Read the model definition and answer for the solid it produces. Units are mm, in the model's axes. Face numbers are marked on the shaded views. A direction names the side the tool comes from. Coordinates: 2 decimals unless noted, no trailing zeros. Write each loop counter-clockwise with the first axis right and the second up, starting at its lowest first coordinate (ties: lowest second). Pieces come first, ordered by that corner, then holes.
(1) Given pin 1 (6.5 mm diameter, centred on x = 13.5, y = 9.5, fed in from +Z); pin 2 (7.5 mm diameter, centred on x = 13, z = 9, fed in from -Y); pin 3 (2 mm diameter, centred on x = 12.5, z = 9.5, fed in from +Y), each flat-ended and moving along its own axis, determine where each tip first touches the part or whether it passes through.
(2) Section C-C on x = 12.5 is taken. Write down the section's boundary in (y, z).
(3) Section D-D on z = 0.5 is taken. Write down the section's boundary in (x, y), then the cut area to 3 significant figures.
(4) Which of the six approach directions +Z, -Z, +X, -X, +Y, -Y give full straight-line access (tool end or side, diameter ignored) to the marked faces 1, 2 and 3?
(5) Section B-B on y = 10.5 is taken. Write down the section's boundary in (x, z).
(6) Find the intervals of material crossed by probe 1 along X at (y, z) = (1.25, 10.5); probe 2 along Y at (x, z) = (7.5, 6); probe 3 along Y at (x, z) = (11.75, 0.5), in increasing order.
(7) Section A-A on z = 7.5 is taken. Write down the section's boundary in (x, y), then the cut area to 3 significant figures.
from build123d import *

# Parameters (mm, degrees)
F0_W      = 22
F0_H      = 15
F1_DEPTH  = 18
F2_T      = -1
F11_DEPTH = 25
F13_DEPTH = 25
F16_R     = 0.5
F17_DEPTH = 50
F20_DEPTH = 50


with BuildPart() as f1:
    # F0 (on Top) → F1 (new body)
    with BuildSketch(Plane.XY):
        with Locations((11, 7.5)):
            Rectangle(F0_W, F0_H)
    extrude(amount=F1_DEPTH)

    # F2
    f2_openings = [f1.faces().sort_by_distance(p)[0] for p in [
        (11, 7.5, 18),
    ]]
    offset(amount=F2_T, openings=f2_openings)

    # F5 (on offset) → F6 section 0
    with BuildSketch(Plane.XY.offset(-2.5)):
        Polygon((-0.5, 2), (-0.5, -0.5), (2, -0.5), (2, 0), (0, 0), (0, 2), align=None)
    # F3 (on face) → F6 section 1
    with BuildSketch(Plane(origin=(0, 0, 0), x_dir=(1, 0, 0), z_dir=(0, 0, -1))):
        Polygon((4, 0), (0, 0), (0, -4), (0.5, -4), (0.5, -0.5), (4, -0.5), align=None)
    loft()

    # F3 (on face) → F7 section 0
    with BuildSketch(Plane(origin=(0, 0, 0), x_dir=(1, 0, 0), z_dir=(0, 0, -1))):
        Polygon((0.5, -11), (0, -11), (0, -15), (4, -15), (4, -14.5), (0.5, -14.5), align=None)
    # F5 (on offset) → F7 section 1
    with BuildSketch(Plane.XY.offset(-2.5)):
        Polygon((-0.5, 13), (0, 13), (0, 15), (2, 15), (2, 15.5), (-0.5, 15.5), align=None)
    loft()

    # F3 (on face) → F8 section 0
    with BuildSketch(Plane(origin=(0, 0, 0), x_dir=(1, 0, 0), z_dir=(0, 0, -1))):
        Polygon((22, -15), (22, -11), (21.5, -11), (21.5, -14.5), (18, -14.5), (18, -15), align=None)
    # F5 (on offset) → F8 section 1
    with BuildSketch(Plane.XY.offset(-2.5)):
        Polygon((20, 15.5), (20, 15), (22, 15), (22, 13), (22.5, 13), (22.5, 15.5), align=None)
    loft()

    # F3 (on face) → F9 section 0
    with BuildSketch(Plane(origin=(0, 0, 0), x_dir=(1, 0, 0), z_dir=(0, 0, -1))):
        Polygon((22, 0), (18, 0), (18, -0.5), (21.5, -0.5), (21.5, -4), (22, -4), align=None)
    # F5 (on offset) → F9 section 1
    with BuildSketch(Plane.XY.offset(-2.5)):
        Polygon((22, 2), (22, 0), (20, 0), (20, -0.5), (22.5, -0.5), (22.5, 2), align=None)
    loft()

    # F10 (on face) → F11 (cut)
    with BuildSketch(Plane.XZ):
        Polygon((20, 15), (22, 15), (22, 18), (0, 18), (0, 15), (2, 15), (3.1547005384, 13), (18.8452994616, 13), align=None)
    extrude(amount=-F11_DEPTH, mode=Mode.SUBTRACT)

    # F12 (on face) → F13 (cut)
    with BuildSketch(Plane.YZ.offset(22)):
        Polygon((13, 15), (2, 15), (3.1547005384, 13), (11.8452994616, 13), align=None)
    extrude(amount=-F13_DEPTH, mode=Mode.SUBTRACT)

    # F16 (on face) → F17 (cut)
    with BuildSketch(Plane(origin=(22.0745514368, 14.8894729496, 0), x_dir=(-0.5591929035, 0.8290375726, 0), z_dir=(0.8290375726, 0.5591929035, 0))):
        with Locations((0.133319712, 14)):
            Circle(F16_R)
    extrude(amount=-F17_DEPTH, mode=Mode.SUBTRACT)

    # F19 (on face) → F20 (cut)
    with BuildSketch(Plane(origin=(15.1206725276, -10.1990224002, 0), x_dir=(0.5591929035, 0.8290375726, 0), z_dir=(0.8290375726, -0.5591929035, 0))):
        with BuildLine():
            ThreePointArc((12.8022438764, 14), (12.6557972669, 14.3535533906), (12.3022438764, 14.5))
            Line((12.3022438764, 14.5), (12.3022438764, 13.5))
            ThreePointArc((12.3022438764, 13.5), (12.6557972669, 13.6464466094), (12.8022438764, 14))
        make_face()
        with BuildLine():
            Line((12.3022438764, 13.5), (12.3022438764, 14.5))
            ThreePointArc((12.3022438764, 14.5), (11.8022438764, 14), (12.3022438764, 13.5))
        make_face()
    extrude(amount=-F20_DEPTH, mode=Mode.SUBTRACT)


solid = f1.part
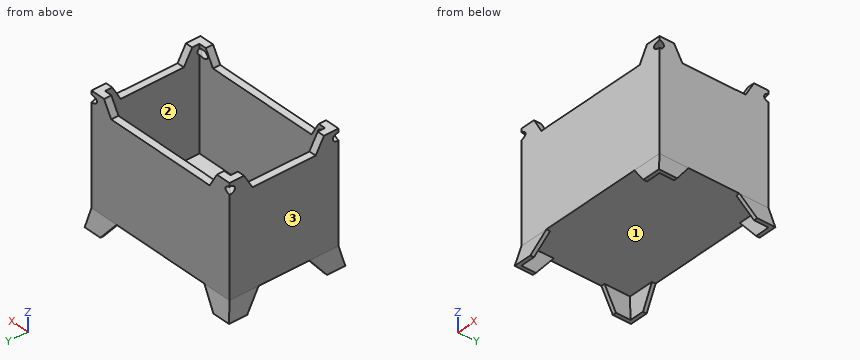
Response:
1. pin 1: stops at z = 1
1. pin 2: stops at y = 0
1. pin 3: stops at y = 15
2. outline: (0, 0) - (15, 0) - (15, 13) - (14, 13) - (14, 1) - (1, 1) - (1, 13) - (0, 13) - close
3. outline: (0, 0) - (22, 0) - (22, 15) - (0, 15) - close
3. area: 330 mm2
4. face 1: -Z
4. face 2: +Z
4. face 3: +Z, -X, +Y, -Y
5. outline: (0, 0) - (22, 0) - (22, 13) - (21, 13) - (21, 1) - (1, 1) - (1, 13) - (0, 13) - close
6. probe 1: x = 0 to 1, 21 to 22
6. probe 2: y = 0 to 1, 14 to 15
6. probe 3: y = 0 to 15
7. outline: (0, 0) - (22, 0) - (22, 15) - (0, 15) - close; hole (1, 1) - (21, 1) - (21, 14) - (1, 14) - close
7. area: 70.0 mm2
